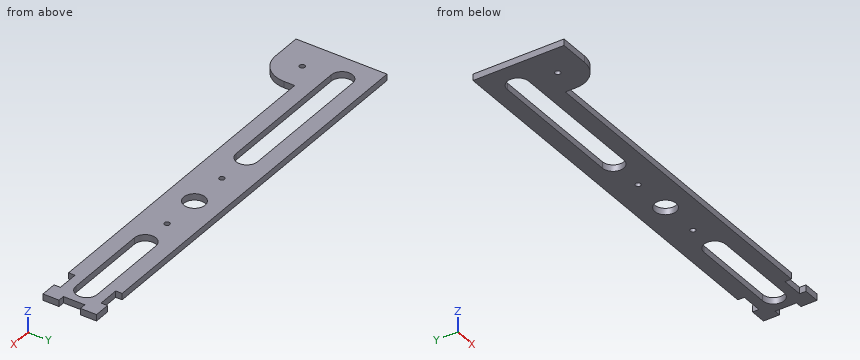
```python
from build123d import *

# Parameters (mm, degrees)
SKETCH1_R           = 2.5
SKETCH1_R_2         = 10
BOSS_EXTRUDE1_DEPTH = 6


with BuildPart() as part:
    # Sketch1 → Boss-Extrude1 (new body)
    with BuildSketch(Plane.XY):
        with BuildLine():
            Line((397.27, -50), (397.27, -35))
            Line((397.27, -35), (391.27, -35))
            Line((391.27, -35), (391.27, -15))
            Line((391.27, -15), (397.27, -15))
            Line((397.27, -15), (397.27, 0))
            Line((397.27, 0), (382.27, 0))
            Line((382.27, 0), (382.27, -6))
            Line((382.27, -6), (362.27, -6))
            Line((362.27, -6), (362.27, 0))
            Line((362.27, 0), (0, 0))
            Line((0, 0), (0, -85))
            Line((0, -85), (28, -85))
            ThreePointArc((28, -85), (45.67766953, -77.67766953), (53, -60))
            Line((53, -60), (53, -50))
            Line((53, -50), (362.27, -50))
            Line((362.27, -50), (362.27, -44))
            Line((362.27, -44), (382.27, -44))
            Line((382.27, -44), (382.27, -50))
            Line((382.27, -50), (397.27, -50))
        make_face()
        with Locations((189.2, -25)):
            Circle(SKETCH1_R, mode=Mode.SUBTRACT)
        with Locations((226.7, -25)):
            Circle(SKETCH1_R_2, mode=Mode.SUBTRACT)
        with Locations((28, -60)):
            Circle(SKETCH1_R, mode=Mode.SUBTRACT)
        with Locations((264.2, -25)):
            Circle(SKETCH1_R, mode=Mode.SUBTRACT)
        with BuildLine():
            Line((25, -35), (155, -35))
            ThreePointArc((155, -35), (165, -25), (155, -15))
            Line((155, -15), (25, -15))
            ThreePointArc((25, -15), (15, -25), (25, -35))
        make_face(mode=Mode.SUBTRACT)
        with BuildLine():
            Line((294.2, -35), (374.2, -35))
            ThreePointArc((374.2, -35), (384.2, -25), (374.2, -15))
            Line((374.2, -15), (294.2, -15))
            ThreePointArc((294.2, -15), (284.2, -25), (294.2, -35))
        make_face(mode=Mode.SUBTRACT)
    extrude(amount=BOSS_EXTRUDE1_DEPTH)


solid = part.part
```
The model under review builds one solid part; all positions refer to its coordinate system, in mm. Round coordinates to 2 decimals unless told otherwise and drop trailing zeros. Order: outer loops, then holes, each group sorted by start corner. A loop starts at its lowest first (then second) coordinate and runs counter-clockwise, first axis right, second up. Notation, with made-up numbers: M 10.25,-15.5 L 50.25,-15.5 A22 ccw 50.25,2.5 Z; hole C -39.5,-14.5 d7. An arc over 180 degrees is marked long. Use a Markdown table: item, result.
1) Insertion check: pin 1 (1.8 mm diameter, centred on x = 222, z = 4.5, fed in from -Y); pin 2 (1.8 mm diameter, centred on y = -3, z = 3, fed in from -X); pin 3 (3 mm diameter, centred on x = 372, z = 4.5, fed in from -Y); pin 4 (1.8 mm diameter, centred on y = -25.5, z = 3.5, fed in from +X). Each pin has a flat end and moves straight along its axis. Give the tip position at first contact, or say it passes through.
Report:
| item | result |
|---|---|
| pin 1 | y = -50 |
| pin 2 | x = 0 |
| pin 3 | y = -44 |
| pin 4 | x = 391.27 |
2) Consider section C-C (y = -74). Write out the cut boundary in (x, z).
Report:
| item | result |
|---|---|
| outline | M 0,0 L 48.71,0 L 48.71,6 L 0,6 Z |
3) Consider section B-B (z = 3.8). Give the number of separate pieces and of enclosed holes in the cut face, then the cut area to 3 significant figures.
Report:
| item | result |
|---|---|
| separate pieces | 1 |
| enclosed holes | 6 |
| area | 16,000 mm^2 |
4) Wall thickness on line 1 along Y through (x, z) = (28, 3.3); line 2 along Y through (x, z) = (226.7, 4.65); line 3 along X through (y, z) = (-22, 5.2): over which ranges is each line inside the solid? List them lowest first. Write a range as [from, to].
Report:
| item | result |
|---|---|
| line 1 | [-85, -62.5], [-57.5, -35], [-15, 0] |
| line 2 | [-50, -35], [-15, 0] |
| line 3 | [0, 15.46], [164.54, 217.16], [236.24, 284.66], [383.74, 391.27] |
5) Consider section A-A (x = 226.7). Write out the cut boundary in (y, z).
Report:
| item | result |
|---|---|
| outline | M -50,0 L -35,0 L -35,6 L -50,6 Z; M -15,0 L 0,0 L 0,6 L -15,6 Z |
